Verification items for the finished model (mm, model axes). Coordinates: 2 decimals unless noted, no trailing zeros. Write each loop counter-clockwise with the first axis right and the second up, starting at its lowest first coordinate (ties: lowest second). Pieces come first, ordered by that corner, then holes. Notation, with made-up numbers: (61, 22) -> (85, 22) arc R36 ccw to (85, 59) -> close; hole circle Ø9 at (-4, -35). An arc over 180 degrees is marked (long way). Write item = value, one per line. Start each with the question number.
(1) Section check A-A (y = 101.5). Record the cut outline in (x, z), plus the area to 3 significant figures.
(2) Material ranges on probe 1 along Y at (x, z) = (0.3, -2.05); probe 2 along X at (y, z) = (-23.5, 0.4); probe 3 along Z at (x, y) = (1.85, 94.5), recorded low to high. Write a range as [from, to].
(3) Gauge pin test, flat end, axial feed: pin 1 Ø1 at (x, y) = (-0.5, 12.5) entering from +Z. Record the tip position at first contact, or that the pin passes through.
```python
from build123d import *

# Parameters (mm, degrees)
SKETCH1_R           = 2.38125
BOSS_EXTRUDE1_DEPTH = 260.35
SKETCH8_W           = 1.6637
SKETCH8_H           = 0.635


with BuildPart() as part:
    # Sketch1 → Boss-Extrude1 (new body, symmetric)
    with BuildSketch(Plane(origin=(0, 0, 0), x_dir=(1, 0, 0), z_dir=(0, 1, 0))):
        Circle(SKETCH1_R)
    extrude(amount=BOSS_EXTRUDE1_DEPTH, both=True)

    # Cut-Sweep1: sweep along a path in Sketch7
    with BuildLine(Plane(origin=(0, -254, 0), x_dir=(-1, 0, 0), z_dir=(0, -1, 0))) as cut_sweep1_path:
        CenterArc((0, 0), 2.38125, 0, 360)
    # Sketch8 → Cut-Sweep1 (sweep, cut)
    with BuildSketch(Plane(origin=(0, 0, 0), x_dir=(0, 0, -1), z_dir=(1, 0, 0))):
        with Locations((2.38125, -254)):
            Rectangle(SKETCH8_W, SKETCH8_H)
    cut_sweep1 = sweep(path=cut_sweep1_path.line, mode=Mode.SUBTRACT)

    # Mirror1: Cut-Sweep1 across plane
    add(cut_sweep1.mirror(Plane.ZX), mode=Mode.SUBTRACT)


solid = part.part
```
Response:
q1.outline = circle Ø4.76 at (0, 0)
q1.area = 17.8 mm2
q2.probe_1 = [-260.35, -254.32], [-253.68, 253.68], [254.32, 260.35]
q2.probe_2 = [-2.35, 2.35]
q2.probe_3 = [-1.5, 1.5]
q3.pin_1 = 2.38
